```python
from build123d import *

# Parameters (mm, degrees)
F1_DEPTH = 2.38125


# Not quite as in the source:
# - a feature names something its author has since deleted; it is built from what else it names


with BuildPart() as f1:
    # F0 (on Top) → F1 (new body)
    with BuildSketch(Plane.XY):
        with BuildLine():
            Line((0.0148852749, -0.0168055587), (-12.9522491515, -11.5022529852))
            Line((-12.9522491515, -11.5022529852), (20.5757791682, -49.3555846081))
            ThreePointArc((20.5757791682, -49.3555846081), (28.7380799657, -53.5635383735), (37.6034379496, -51.168656953))
            ThreePointArc((37.6034379496, -51.168656953), (39.8947610083, -49.4030165485), (42.1032952287, -47.5348559574))
            Line((42.1032952287, -47.5348559574), (32.0658696462, -36.2025462971))
            ThreePointArc((32.0658696462, -36.2025462971), (22.9586334857, -35.6506997271), (23.5104800557, -26.5434635666))
            Line((23.5104800557, -26.5434635666), (0.0148852749, -0.0168055587))
        make_face()
        with BuildLine():
            Line((12.9820197013, 11.4686418678), (0.0148852749, -0.0168055587))
            Line((0.0148852749, -0.0168055587), (23.5104800557, -26.5434635666))
            ThreePointArc((23.5104800557, -26.5434635666), (30.4363031351, -25.4899309777), (34.2397748509, -31.3730049319))
            ThreePointArc((34.2397748509, -31.3730049319), (33.6712488051, -34.0211332161), (32.0658696462, -36.2025462971))
            Line((32.0658696462, -36.2025462971), (42.1032952287, -47.5348559574))
            ThreePointArc((42.1032952287, -47.5348559574), (44.2244575032, -45.5680519503), (46.2538460369, -43.5066860011))
            ThreePointArc((46.2538460369, -43.5066860011), (49.7016552964, -34.9953617498), (46.510048021, -26.3846897551))
            Line((46.510048021, -26.3846897551), (12.9820197013, 11.4686418678))
        make_face()
        with BuildLine():
            Line((-48.3172110137, 28.4249868882), (-12.9522491515, -11.5022529852))
            Line((-12.9522491515, -11.5022529852), (0.0148852749, -0.0168055587))
            Line((0.0148852749, -0.0168055587), (0, 0))
            Line((0, 0), (-24.3525459603, 27.4941606857))
            ThreePointArc((-24.3525459603, 27.4941606857), (-33.4597821208, 28.0460072558), (-32.9079355507, 37.1532434163))
            Line((-32.9079355507, 37.1532434163), (-44.6294929424, 50.3869473148))
            Line((-44.6294929424, 50.3869473148), (-49.0520937641, 44.3552682835))
            ThreePointArc((-49.0520937641, 44.3552682835), (-51.4967480049, 36.2604022841), (-48.3172110137, 28.4249868882))
        make_face()
        with BuildLine():
            Line((0, 0), (0.0148852749, -0.0168055587))
            Line((0.0148852749, -0.0168055587), (12.9820197013, 11.4686418678))
            Line((12.9820197013, 11.4686418678), (-22.3829421609, 51.3958817412))
            ThreePointArc((-22.3829421609, 51.3958817412), (-29.7771159339, 55.4982449772), (-38.1079364614, 54.0488936593))
            Line((-38.1079364614, 54.0488936593), (-44.6294929424, 50.3869473148))
            Line((-44.6294929424, 50.3869473148), (-32.9079355507, 37.1532434163))
            ThreePointArc((-32.9079355507, 37.1532434163), (-25.9821124713, 38.2067760052), (-22.1786407555, 32.323702051))
            ThreePointArc((-22.1786407555, 32.323702051), (-22.7471668013, 29.6755737668), (-24.3525459603, 27.4941606857))
            Line((-24.3525459603, 27.4941606857), (0, 0))
        make_face()
    extrude(amount=F1_DEPTH)


solid = f1.part
```
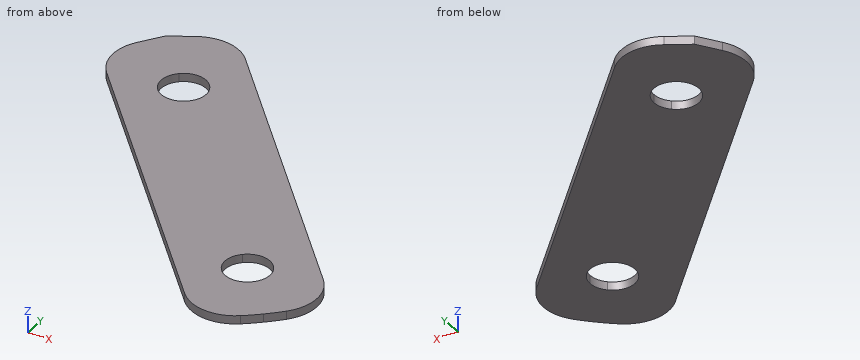
The model under review builds one solid part; all positions refer to its coordinate system, in mm. Round coordinates to 2 decimals unless told otherwise and drop trailing zeros. Write each loop counter-clockwise with the first axis right and the second up, starting at its lowest first coordinate (ties: lowest second). Pieces come first, ordered by that corner, then holes. Notation, with made-up numbers: (16, -22) - (59, -22) arc R17 cw to (59, -18) - close; hole circle Ø5 at (84.25, 10.5). An arc over 180 degrees is marked (long way). Answer as CSV lines item,"result". Start each with the question number.
(1) We need section C-C on x = -7. State the section outline as (y, z) points, plus the area to 3 significant figures.
(2) We need section D-D on y = -21. State the section outline as (x, z) points, plus the area to 3 significant figures.
(3) We need section B-B on x = -30.5. State the section outline as (y, z) points, plus the area to 3 significant figures.
(4) To check wall thickness, follow line 1 (X direction, y = -37, z = 0.8); line 2 (Y direction, x = -32.5, z = 0.3); line 3 (Y direction, x = 30, z = 0.5). State the ranges of each line that lie inside material, in increasing order.
(5) We need section A-A on z = 1.55. State the section outline as (x, y) points, plus the area to 3 significant figures.
Worked answers:
1,outline,"(-18.22, 0) - (34.03, 0) - (34.03, 2.38) - (-18.22, 2.38) - close"
1,area,"124 mm²"
2,outline,"(-4.54, 0) - (41.74, 0) - (41.74, 2.38) - (-4.54, 2.38) - close"
2,area,"110 mm²"
3,outline,"(8.31, 0) - (26.15, 0) - (26.15, 2.38) - (8.31, 2.38) - close; (38.5, 0) - (55.6, 0) - (55.6, 2.38) - (38.5, 2.38) - close"
3,area,"83.2 mm²"
4,line 1,"9.63 to 24.63, 30.94 to 49.51"
4,line 2,"10.57 to 27.16, 37.49 to 55.66"
4,line 3,"-53.63 to -37.43, -25.31 to -7.74"
5,outline,"(-49.05, 44.36) arc R12.7 ccw to (-48.32, 28.42) - (20.58, -49.36) arc R12.7 ccw to (37.6, -51.17) arc R63.5 ccw to (46.25, -43.51) arc R12.7 ccw to (46.51, -26.38) - (-22.38, 51.4) arc R12.7 ccw to (-38.11, 54.05) - (-44.63, 50.39) - close; hole circle Ø12.9 at (-28.63, 32.32); hole circle Ø12.9 at (27.79, -31.37)"
5,area,"4,090 mm²"
